Design review of the part built by this model. Coordinates are the model's own, in mm. Face numbers are marked on the shaded views. A direction names the side the tool comes from. Give positions to 0.01 mm unless a question says otherwise; leave off trailing zeros. Loops run counter-clockwise (first coordinate to the right, second up) from the corner with the lowest first, then second, coordinate; pieces in that order, holes last.
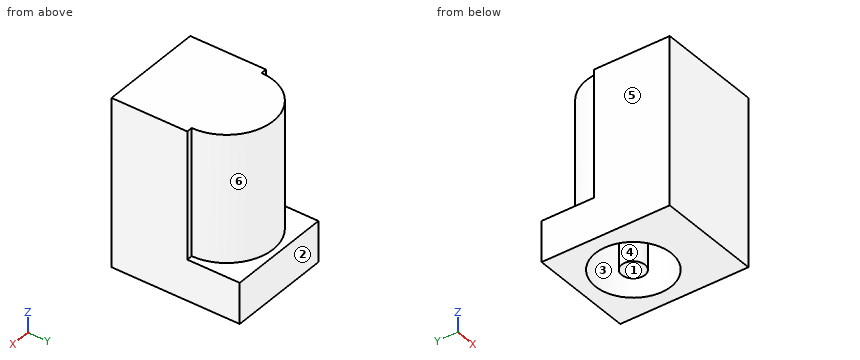
from build123d import *

# Parameters (mm, degrees)
SKETCH1_W           = 9
SKETCH1_H           = 11
BOSS_EXTRUDE1_DEPTH = 3.5
BOSS_EXTRUDE2_DEPTH = 14.4
SKETCH3_R           = 3.25
SKETCH3_R_2         = 1
CUT_EXTRUDE1_DEPTH  = 10


with BuildPart() as part:
    # Sketch1 → Boss-Extrude1 (new body)
    with BuildSketch(Plane.XY):
        with Locations((4.5, 5.5)):
            Rectangle(SKETCH1_W, SKETCH1_H)
    extrude(amount=BOSS_EXTRUDE1_DEPTH)

    # Sketch2 → Boss-Extrude2 (add)
    with BuildSketch(Plane(origin=(0, 0, 0), x_dir=(-1, 0, 0), z_dir=(0, 0, -1))):
        with BuildLine():
            Line((-0.5, 6.5), (0, 6.5))
            Line((0, 6.5), (0, 0))
            Line((0, 0), (-9, 0))
            Line((-9, 0), (-9, 6.5))
            Line((-9, 6.5), (-8.5, 6.5))
            ThreePointArc((-8.5, 6.5), (-4.5, 10.5), (-0.5, 6.5))
        make_face()
    extrude(amount=-BOSS_EXTRUDE2_DEPTH)

    # Sketch3 → Cut-Extrude1 (cut)
    with BuildSketch(Plane(origin=(0, 0, 0), x_dir=(-1, 0, 0), z_dir=(0, 0, -1))):
        with Locations((-4.5, 6.5)):
            Circle(SKETCH3_R)
        with Locations((-4.5, 6.5)):
            Circle(SKETCH3_R_2, mode=Mode.SUBTRACT)
    extrude(amount=-CUT_EXTRUDE1_DEPTH, mode=Mode.SUBTRACT)


solid = part.part
Q1. Insertion check: pin 1 (1.5 mm diameter, centred on y = 7.5, z = 6, fed in from -X); pin 2 (2 mm diameter, centred on x = 1, z = 8.5, fed in from +Y); pin 3 (1 mm diameter, centred on x = 7.5, y = 3, fed in from -Z). Each pin has a flat end and moves straight along its axis. Give the tip position at first contact, or say it passes through.
Results:
pin 1: stops at x = 0.51
pin 2: stops at y = 9.62
pin 3: stops at z = 0
Q2. Wall thickness on line 1 (Y direction, x = 4.5, z = 3); line 2 (Y direction, x = 4.5, z = 4.75); line 3 (Y direction, x = 3, z = 1.25): over which ranges is each line inside the solid? List them lowest first.
Results:
line 1: y = 0 to 3.25, 5.5 to 7.5, 9.75 to 11
line 2: y = 0 to 3.25, 5.5 to 7.5, 9.75 to 10.5
line 3: y = 0 to 3.62, 9.38 to 11
Q3. Take a section at B-B (x = 4.5). Give the boundary of the cut face in (y, z), plus the area to 3 significant figures.
Results:
outline: (0, 0) - (3.25, 0) - (3.25, 10) - (5.5, 10) - (5.5, 0) - (7.5, 0) - (7.5, 10) - (9.75, 10) - (9.75, 0) - (11, 0) - (11, 3.5) - (10.5, 3.5) - (10.5, 14.4) - (0, 14.4) - close
area: 108 mm2
Q4. Tool access review of the marked faces 4, 5 and 6: name each direction out of +Z, -Z, +X, -X, +Y, -Y from which nothing blocks a thin tool from reaching the whole face with its end or side.
Results:
face 4: -Z
face 5: +Z, -Z, -X, +Y, -Y
face 6: +Z, +Y
Q5. Take a section at C-C (y = 10). Give the boundary of the cut face in (x, z).
Results:
outline: (0, 0) - (9, 0) - (9, 3.5) - (6.44, 3.5) - (6.44, 14.4) - (2.56, 14.4) - (2.56, 3.5) - (0, 3.5) - close
Q6. Take a section at A-A (z = 6.75). Give the boundary of the cut face in (x, y).
Results:
outline: (0, 0) - (9, 0) - (9, 6.5) - (8.5, 6.5) arc R4 ccw to (0.5, 6.5) - (0, 6.5) - close; circle Ø2 at (4.5, 6.5); hole circle Ø6.5 at (4.5, 6.5)
Q7. Draft analysis for pull direction Y (two halves, no side actions). For the marked faces 1, 2 and 3, state which applies: pulls with the +Y half, pulls with the -Y half, needs draft (parallel to the pull), parting line crosses it, or undercut.
Results:
face 1: needs draft
face 2: pulls with the +Y half
face 3: undercut
Q8. Take a section at D-D (x = 7.25). Give the boundary of the cut face in (y, z), plus the area to 3 significant figures.
Results:
outline: (0, 0) - (4.77, 0) - (4.77, 10) - (8.23, 10) - (8.23, 0) - (11, 0) - (11, 3.5) - (9.4, 3.5) - (9.4, 14.4) - (0, 14.4) - close
area: 106 mm2
